Source: CAD feature listing. Evaluate the final solid. Frame: model axes, mm. Face numbers are marked on the shaded views. A direction names the side the tool comes from. Give positions to 0.01 mm unless a question says otherwise; leave off trailing zeros. Loops run counter-clockwise (first coordinate to the right, second up) from the corner with the lowest first, then second, coordinate; pieces in that order, holes last. Notation, with made-up numbers: M -29.75,53 L 4.25,53 A8 ccw 4.25,64 Z; hole C 75.5,-23.5 d3. An arc over 180 degrees is marked long. Put each result on its own line as item: value. Start each with the question number.
```python
from build123d import *

# Parameters (mm, degrees)
SKETCH1_R           = 75
BOSS_EXTRUDE1_DEPTH = 30
SKETCH2_R           = 75
SKETCH2_R_2         = 7.5
CUT_EXTRUDE1_DEPTH  = 20
SKETCH3_R           = 2.5
CUT_EXTRUDE2_DEPTH  = 30
SKETCH4_R           = 2.5
CUT_EXTRUDE3_DEPTH  = 10


with BuildPart() as part:
    # Sketch1 → Boss-Extrude1 (new body)
    with BuildSketch(Plane(origin=(0, 0, 0), x_dir=(1, 0, 0), z_dir=(0, 1, 0))):
        with Locations(Location((0, 0, 0), (0, 0, 270))):
            Circle(SKETCH1_R)
    extrude(amount=BOSS_EXTRUDE1_DEPTH)

    # Sketch2 → Cut-Extrude1 (cut)
    with BuildSketch(Plane.XZ):
        with Locations(Location((0, 0, 0), (0, 0, 270))):
            Circle(SKETCH2_R)
        with Locations(Location((0, 0, 0), (0, 0, 270))):
            Circle(SKETCH2_R_2, mode=Mode.SUBTRACT)
    extrude(amount=-CUT_EXTRUDE1_DEPTH, mode=Mode.SUBTRACT)

    # Sketch3 → Cut-Extrude2 (cut)
    with BuildSketch(Plane(origin=(0, 30, 0), x_dir=(1, 0, 0), z_dir=(0, 1, 0))):
        with Locations(Location((0, 0, 0), (0, 0, 270))):
            Circle(SKETCH3_R)
    extrude(amount=-CUT_EXTRUDE2_DEPTH, mode=Mode.SUBTRACT)

    # Sketch4 → Cut-Extrude3 (cut)
    with BuildSketch(Plane(origin=(0, 30, 0), x_dir=(1, 0, 0), z_dir=(0, 1, 0))):
        with Locations(Location((-15, 20, 0), (0, 0, 270))):
            Circle(SKETCH4_R)
        with Locations(Location((15, 20, 0), (0, 0, 270))):
            Circle(SKETCH4_R)
        with Locations(Location((-15, -20, 0), (0, 0, 270))):
            Circle(SKETCH4_R)
        with Locations(Location((15, -20, 0), (0, 0, 270))):
            Circle(SKETCH4_R)
    extrude(amount=-CUT_EXTRUDE3_DEPTH, mode=Mode.SUBTRACT)


solid = part.part
```
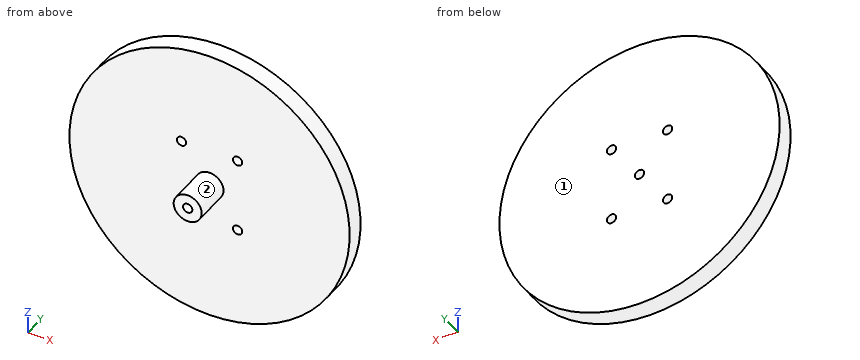
1. Set-up query: the marked faces 1 and 2. Return all of +Z, -Z, +X, -X, +Y, -Y with unobstructed straight access to the full face (end or side cutting, diameter ignored); none if empty.
2. Ray query, line 1 (X direction, y = 26.75, z = -20); line 2 (X direction, y = 18.25, z = 0); line 3 (Y direction, x = -15.5, z = 54). Return the intervals inside material, ascending.
3. Section B-B, the plane x = 0. Output: boundary loops of the cut face in (y, z).
4. Section C-C, the plane y = 22. Output: boundary loops of the cut face in (x, z), plus the area to 3 significant figures.
5. Contact query for flat-ended pins moving along their axis: pin 1 (2 mm diameter, centred on x = 38.5, y = 27, fed in from -Z); pin 2 (12 mm diameter, centred on x = 17.5, y = 23.5, fed in from +Z); pin 3 (6 mm diameter, centred on x = -15, z = 20, fed in from -Y). Output: stop coordinate, or through.
6. Section D-D, the plane x = -15. Output: boundary loops of the cut face in (y, z).
7. Section A-A, the plane z = 0. Output: boundary loops of the cut face in (x, y), plus the area to 3 significant figures.
Results found:
1. face 1: +Z, -Z, +X, -X, +Y
1. face 2: -Y
2. line 1: -72.28 to -17.5, -12.5 to 12.5, 17.5 to 72.28
2. line 2: -7.5 to -2.5, 2.5 to 7.5
2. line 3: 20 to 30
3. outline: M 0,-7.5 L 20,-7.5 L 20,-75 L 30,-75 L 30,-2.5 L 0,-2.5 Z; M 0,2.5 L 30,2.5 L 30,75 L 20,75 L 20,7.5 L 0,7.5 Z
4. outline: C 0,0 d150; hole C -15,-20 d5; hole C -15,20 d5; hole C 0,0 d5; hole C 15,-20 d5; hole C 15,20 d5
4. area: 17,600 mm²
5. pin 1: z = -64.95
5. pin 2: z = 74.11
5. pin 3: y = 20
6. outline: M 20,-73.48 L 30,-73.48 L 30,-22.5 L 20,-22.5 Z; M 20,-17.5 L 30,-17.5 L 30,17.5 L 20,17.5 Z; M 20,22.5 L 30,22.5 L 30,73.48 L 20,73.48 Z
7. outline: M -75,20 L -7.5,20 L -7.5,0 L -2.5,0 L -2.5,30 L -75,30 Z; M 2.5,0 L 7.5,0 L 7.5,20 L 75,20 L 75,30 L 2.5,30 Z
7. area: 1,650 mm²
